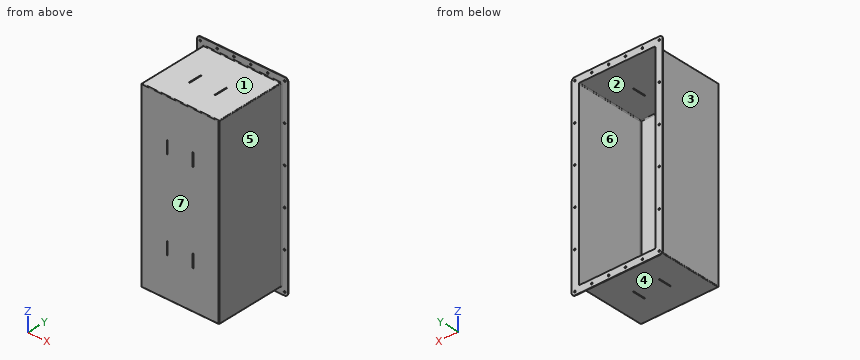
from build123d import *

# Parameters (mm, degrees)
SKETCH1_W              = 226.478396166
SKETCH1_H              = 526.585680888
CONTAINER_BOTTOM_DEPTH = 2.2098
SKETCH2_W              = 226.478396166
SKETCH2_H              = 526.585680888
SKETCH2_W_2            = 222.942716166
SKETCH2_H_2            = 523.050000888
CONTAINER_WALLS_DEPTH  = 203.2
SKETCH64_W             = 264.578396166
SKETCH64_H             = 564.685680888
SKETCH64_W_2           = 226.478396166
SKETCH64_H_2           = 526.585680888
BOSS_EXTRUDE3_DEPTH    = 1.76784
F_10_CLEARANCE_HOLE1_D = 4.9784
FILLET1_R              = 2.54
CUT_EXTRUDE1_REACH     = 375.378
SKETCH42_W             = 2.56159
SKETCH42_H             = 38.1
LPATTERN1_COUNT        = 2
LPATTERN1_PITCH        = 74.903518722
LPATTERN1_COUNT_DIR2   = 2
LPATTERN1_PITCH_DIR2   = 261.525000444
SKETCH43_W             = 2.56159
SKETCH43_H             = 38.1
CUT_EXTRUDE2_DEPTH     = 598.839371507
LPATTERN2_COUNT        = 2
LPATTERN2_PITCH        = 74.903518722
FILLET2_R              = 2
FILLET3_R              = 9.525


with BuildPart() as part:
    # Sketch1 → Container_Bottom (new body)
    with BuildSketch(Plane(origin=(0, 0, 0), x_dir=(1, 0, 0), z_dir=(0, 1, 0))):
        Rectangle(SKETCH1_W, SKETCH1_H)
    extrude(amount=CONTAINER_BOTTOM_DEPTH)

    # Sketch2 → Container_Walls (add)
    with BuildSketch(Plane(origin=(0, 2.2098, 0), x_dir=(1, 0, 0), z_dir=(0, 1, 0))):
        Rectangle(SKETCH2_W, SKETCH2_H)
        Rectangle(SKETCH2_W_2, SKETCH2_H_2, mode=Mode.SUBTRACT)
    extrude(amount=CONTAINER_WALLS_DEPTH)

    # Sketch64 → Boss-Extrude3 (add)
    with BuildSketch(Plane(origin=(0, 205.4098, 0), x_dir=(1, 0, 0), z_dir=(0, 1, 0))):
        Rectangle(SKETCH64_W, SKETCH64_H)
        Rectangle(SKETCH64_W_2, SKETCH64_H_2, mode=Mode.SUBTRACT)
    extrude(amount=-BOSS_EXTRUDE3_DEPTH)

    # #10 Clearance Hole1 (through all)
    with Locations(Plane(origin=(0, 205.4098, 0), x_dir=(1, 0, 0), z_dir=(0, 1, 0))):
        with Locations((-122.764198083, 272.817840444), (-122.764198083, 163.690704266), (-122.764198083, 54.563568089), (-122.764198083, -54.563568089), (-122.764198083, -163.690704266), (-122.764198083, -272.817840444), (-73.65851885, -272.817840444), (-24.552839617, -272.817840444), (-73.65851885, 272.817840444), (-24.552839617, 272.817840444)):
            f_10_clearance_hole1 = Hole(F_10_CLEARANCE_HOLE1_D / 2)

    # Mirror3: #10 Clearance Hole1 across plane
    add(f_10_clearance_hole1.mirror(Plane(origin=(0, 0, 0), x_dir=(0, 0, 1), z_dir=(1, 0, 0))), mode=Mode.SUBTRACT)

    # Fillet1
    fillet1_edges = [part.edges().sort_by_distance(p)[0] for p in [
        (-111.471358083, 2.2098, 0),
        (0, 2.2098, 261.525000444),
        (111.471358083, 2.2098, 0),
        (0, 2.2098, -261.525000444),
        (-111.471358083, 103.8098, 261.525000444),
        (111.471358083, 103.8098, 261.525000444),
        (111.471358083, 103.8098, -261.525000444),
        (-111.471358083, 103.8098, -261.525000444),
    ]]
    fillet(fillet1_edges, radius=FILLET1_R)

    # Sketch42 → Cut-Extrude1 (cut, up to next)
    with BuildSketch(Plane.XZ, mode=Mode.PRIVATE) as cut_extrude1_sk1:
        with Locations((-37.451759361, 130.762500222)):
            Rectangle(SKETCH42_W, SKETCH42_H)
    cut_extrude1_tool1 = extrude(cut_extrude1_sk1.sketch, amount=-CUT_EXTRUDE1_REACH, mode=Mode.PRIVATE) & part.part
    cut_extrude1 = cut_extrude1_tool1.solids().sort_by_distance((-37.451759, 0, 130.7625))[0]
    add(cut_extrude1, mode=Mode.SUBTRACT)

    # LPattern1: Cut-Extrude1 2 × 2
    with Locations(*[(i * LPATTERN1_PITCH, 0, -j * LPATTERN1_PITCH_DIR2) for i in range(LPATTERN1_COUNT) for j in range(LPATTERN1_COUNT_DIR2) if (i, j) != (0, 0)]):
        add(cut_extrude1, mode=Mode.SUBTRACT)

    # Sketch43 → Cut-Extrude2 (cut, through all)
    with BuildSketch(Plane(origin=(0, 0, -263.292840444), x_dir=(-1, 0, 0), z_dir=(0, 0, -1))):
        with Locations((-37.451759361, 91.1098)):
            Rectangle(SKETCH43_W, SKETCH43_H)
    cut_extrude2 = extrude(amount=-CUT_EXTRUDE2_DEPTH, mode=Mode.SUBTRACT)

    # LPattern2: Cut-Extrude2 ×2
    with Locations(*[(-i * LPATTERN2_PITCH, 0, 0) for i in range(1, LPATTERN2_COUNT)]):
        add(cut_extrude2, mode=Mode.SUBTRACT)

    # Fillet2
    fillet2_edges = [part.edges().sort_by_distance(p)[0] for p in [
        (-113.239198083, 101.82098, -263.292840444),
        (113.239198083, 101.82098, -263.292840444),
        (113.239198083, 101.82098, 263.292840444),
        (-113.239198083, 101.82098, 263.292840444),
        (0, 203.64196, -263.292840444),
        (-113.239198083, 203.64196, 0),
        (0, 203.64196, 263.292840444),
        (113.239198083, 203.64196, 0),
        (0, 0, -263.292840444),
        (113.239198083, 0, 0),
        (0, 0, 263.292840444),
        (-113.239198083, 0, 0),
    ]]
    fillet(fillet2_edges, radius=FILLET2_R)

    # Fillet3
    fillet3_edges = [part.edges().sort_by_distance(p)[0] for p in [
        (-132.289198083, 204.52588, 282.342840444),
        (-132.289198083, 204.52588, -282.342840444),
        (132.289198083, 204.52588, -282.342840444),
        (132.289198083, 204.52588, 282.342840444),
    ]]
    fillet(fillet3_edges, radius=FILLET3_R)


solid = part.part
Build history of the part. All positions in model axes, mm. Face numbers are marked on the shaded views. A direction names the side the tool comes from. Give positions to 0.01 mm unless a question says otherwise; leave off trailing zeros. Loops run counter-clockwise (first coordinate to the right, second up) from the corner with the lowest first, then second, coordinate; pieces in that order, holes last. Notation, with made-up numbers: (68.5, -20.5) -> (72.5, -20.5) arc R17 ccw to (72.5, 5.5) -> close; hole circle Ø7 at (36, 73). An arc over 180 degrees is marked (long way). Answer in a Markdown table with one row per item.
Item 1: Slice it at D-D on x = -92.5. Write the cut outline in (y, z) (3 decimals).
Findings below:
| item | result |
|---|---|
| outline | (0, -261.293) arc R2 ccw to (2, -263.293) -> (201.642, -263.293) arc R2 cw to (203.642, -265.293) -> (203.642, -282.343) -> (205.41, -282.343) -> (205.41, -261.525) -> (4.75, -261.525) arc R2.54 cw to (2.21, -258.985) -> (2.21, 258.985) arc R2.54 cw to (4.75, 261.525) -> (205.41, 261.525) -> (205.41, 282.343) -> (203.642, 282.343) -> (203.642, 265.293) arc R2 cw to (201.642, 263.293) -> (2, 263.293) arc R2 ccw to (0, 261.293) -> close |
Item 2: Slice it at C-C on z = 77. Write the cut outline in (x, y).
Findings below:
| item | result |
|---|---|
| outline | (-132.29, 203.64) -> (-115.24, 203.64) arc R2 cw to (-113.24, 201.64) -> (-113.24, 2) arc R2 ccw to (-111.24, 0) -> (111.24, 0) arc R2 ccw to (113.24, 2) -> (113.24, 201.64) arc R2 cw to (115.24, 203.64) -> (132.29, 203.64) -> (132.29, 205.41) -> (111.47, 205.41) -> (111.47, 4.75) arc R2.54 cw to (108.93, 2.21) -> (-108.93, 2.21) arc R2.54 cw to (-111.47, 4.75) -> (-111.47, 205.41) -> (-132.29, 205.41) -> close |
Item 3: Probe line 1 along Z through (x, y) = (-72.5, 134) (3 decimals); line 2 along X through (y, z) = (23.5, 57); line 3 along Y through (x, z) = (15.5, -157.5). List the from-to ranges inside material, lowest first. Write a range as [from, to].
Findings below:
| item | result |
|---|---|
| line 1 | z = [-263.293, -261.525], [261.525, 263.293] |
| line 2 | x = [-113.24, -111.47], [111.47, 113.24] |
| line 3 | y = [0, 2.21] |
Item 4: Slice it at A-A on y = 86.5. Give the number of separate pieces and of enclosed holes in the cut face, plus the area to 3 significant figures.
Findings below:
| item | result |
|---|---|
| separate pieces | 4 |
| enclosed holes | 0 |
| area | 2,630 mm² |
Item 5: Flat gauge pins, fed straight in: P1, Ø1.8, axis at x = 38, y = 1, coming from the +Z side; P2, Ø0.9, axis at x = 37, z = 262.5, coming from the -Y side; P3, Ø4, axis at x = -122.76, z = -163.69, coming from the +Y side; P4, Ø3, axis at y = 82.5, z = 118.5, coming from the +X side. Where does each tip first touch, or does it go through?
Findings below:
| item | result |
|---|---|
| P1 | stops at z = 263.29 |
| P2 | stops at y = 0.15 |
| P3 | passes through |
| P4 | stops at x = 113.24 |
Item 6: Mould opens along X. For the marked faces 1, 2 and 3 say: pulls with the +X half, pulls with the -X half, needs draft (parallel to the pull), parting line crosses it, or undercut.
Findings below:
| item | result |
|---|---|
| face 1 | needs draft |
| face 2 | undercut |
| face 3 | pulls with the -X half |
Item 7: Tool access for the marked faces 4, 5, 6 and 7: list every direction of +Z, -Z, +X, -X, +Y, -Y with a clear straight run to the whole face (end or side of a thin tool).
Findings below:
| item | result |
|---|---|
| face 4 | -Z, +X, -X, -Y |
| face 5 | +Z, -Z, +X, -Y |
| face 6 | +Y |
| face 7 | +Z, -Z, +X, -X, -Y |
Item 8: Slice it at B-B on y = 34. Write the cut outline in (x, z) (3 decimals), plus the area to 3 significant figures.
Findings below:
| item | result |
|---|---|
| outline | (-113.239, -261.293) arc R2 ccw to (-111.239, -263.293) -> (111.239, -263.293) arc R2 ccw to (113.239, -261.293) -> (113.239, 261.293) arc R2 ccw to (111.239, 263.293) -> (-111.239, 263.293) arc R2 ccw to (-113.239, 261.293) -> close; hole (-111.471, -258.985) arc R2.54 ccw to (-108.931, -261.525) -> (108.931, -261.525) arc R2.54 ccw to (111.471, -258.985) -> (111.471, 258.985) arc R2.54 ccw to (108.931, 261.525) -> (-108.931, 261.525) arc R2.54 ccw to (-111.471, 258.985) -> close |
| area | 2,650 mm² |
